```python
from build123d import *

# Parameters (mm, degrees)
SKETCH1_W           = 177.8
SKETCH1_H           = 63.5
SKETCH1_R           = 2.032
BOSS_EXTRUDE1_DEPTH = 6.35
CUT_EXTRUDE1_DEPTH  = 6.35
SKETCH3_R           = 2.413
CUT_EXTRUDE2_DEPTH  = 6.35
LPATTERN1_COUNT     = 3
LPATTERN1_PITCH     = 12.7


with BuildPart() as part:
    # Sketch1 → Boss-Extrude1 (new body)
    with BuildSketch(Plane.XY):
        Rectangle(SKETCH1_W, SKETCH1_H)
        with Locations((-82.804, 25.654)):
            Circle(SKETCH1_R, mode=Mode.SUBTRACT)
        with Locations((-82.804, 0)):
            Circle(SKETCH1_R, mode=Mode.SUBTRACT)
        with Locations((-82.804, -25.654)):
            Circle(SKETCH1_R, mode=Mode.SUBTRACT)
        with Locations((82.804, -25.654)):
            Circle(SKETCH1_R, mode=Mode.SUBTRACT)
        with Locations((82.804, 0)):
            Circle(SKETCH1_R, mode=Mode.SUBTRACT)
        with Locations((82.804, 25.654)):
            Circle(SKETCH1_R, mode=Mode.SUBTRACT)
    extrude(amount=BOSS_EXTRUDE1_DEPTH)

    # Sketch2 → Cut-Extrude1 (cut)
    with BuildSketch(Plane.XY.offset(6.35)):
        Polygon((-75.063183589, 28.589529071), (-75.063183589, -27.290470929), (-51.281087561, -27.290470929), (-50.94437734, 0.649529071), (-50.94437734, 28.589529071), align=None)
        Polygon((-50.94437734, 0.649529071), (-51.281087561, -27.290470929), (-7.031936064, -27.290470929), (-7.031936064, 28.589529071), (-50.94437734, 28.589529071), align=None)
    extrude(amount=-CUT_EXTRUDE1_DEPTH, mode=Mode.SUBTRACT)

    # Sketch3 → Cut-Extrude2 (cut)
    with BuildSketch(Plane.XY.offset(6.35)):
        with Locations((63.5, 19.05)):
            Circle(SKETCH3_R)
    cut_extrude2 = extrude(amount=-CUT_EXTRUDE2_DEPTH, mode=Mode.SUBTRACT)

    # LPattern1: Cut-Extrude2 ×3
    with Locations(*[(0, -i * LPATTERN1_PITCH, 0) for i in range(1, LPATTERN1_COUNT)]):
        add(cut_extrude2, mode=Mode.SUBTRACT)


solid = part.part
```
Geometry: final body of the model. Coordinates: model frame, mm. A direction names the side the tool comes from. Coordinates: 2 decimals unless noted, no trailing zeros. Order: outer loops, then holes, each group sorted by start corner. A loop starts at its lowest first (then second) coordinate and runs counter-clockwise, first axis right, second up. Notation, with made-up numbers: (22.25, -27.75) - (72.25, -27.75) arc R33 cw to (72.25, 3.25) - close; hole circle Ø11 at (0.25, 85.25). An arc over 180 degrees is marked (long way). Write each question's results on one line, items separated by ' | '.
1) Section A-A, the plane y = 19.05. Return loops of the section in (x, z), plus the area to 3 significant figures.
Results list:
outline: (-88.9, 0) - (-75.06, 0) - (-75.06, 6.35) - (-88.9, 6.35) - close; (-7.03, 0) - (61.09, 0) - (61.09, 6.35) - (-7.03, 6.35) - close; (65.91, 0) - (88.9, 0) - (88.9, 6.35) - (65.91, 6.35) - close | area: 666 mm^2
2) Section B-B, the plane x = 63.5. Return loops of the section in (y, z).
Results list:
outline: (-31.75, 0) - (-8.76, 0) - (-8.76, 6.35) - (-31.75, 6.35) - close; (-3.94, 0) - (3.94, 0) - (3.94, 6.35) - (-3.94, 6.35) - close; (8.76, 0) - (16.64, 0) - (16.64, 6.35) - (8.76, 6.35) - close; (21.46, 0) - (31.75, 0) - (31.75, 6.35) - (21.46, 6.35) - close
3) Set-up query: faces 1 (the flat face through (19, 0, 6.35)), 2 (the flat face through (-41, 28.59, 3)). Return all of +Z, -Z, +X, -X, +Y, -Y with unobstructed straight access to the full face (end or side cutting, diameter ignored); none if empty.
Results list:
face 1: +Z, +X, -X, +Y, -Y | face 2: +Z, -Z
4) Pull-direction query (X, two-part tool) for faces 3 (the flat face through (88.9, 0, 3)), 4 (the flat face through (19, 0, 0)), 5 (the flat face through (-88.9, 0, 3)), 6 (the cylindrical face through (61.09, 6.46, 3.22)); classes: pulls with the +X half, pulls with the -X half, needs draft (parallel to the pull), parting line crosses it, or undercut.
Results list:
face 3: pulls with the +X half | face 4: needs draft | face 5: pulls with the -X half | face 6: undercut
5) Line query: line 1 (X direction, y = 19, z = 3.25); line 2 (Y direction, x = 63.5, z = 4.5); line 3 (Y direction, x = -23, z = 1.5). Output: solid intervals per line, ascending. Write a range as from..to.
Results list:
line 1: -88.9..-75.06, -7.03..61.09, 65.91..88.9 | line 2: -31.75..-8.76, -3.94..3.94, 8.76..16.64, 21.46..31.75 | line 3: -31.75..-27.29, 28.59..31.75
6) Section D-D, the plane x = -46. Return loops of the section in (y, z), plus the area to 3 significant figures.
Results list:
outline: (-31.75, 0) - (-27.29, 0) - (-27.29, 6.35) - (-31.75, 6.35) - close; (28.59, 0) - (31.75, 0) - (31.75, 6.35) - (28.59, 6.35) - close | area: 48.4 mm^2
7) Section C-C, the plane y = -15.5. Return loops of the section in (x, z).
Results list:
outline: (-88.9, 0) - (-75.06, 0) - (-75.06, 6.35) - (-88.9, 6.35) - close; (-7.03, 0) - (88.9, 0) - (88.9, 6.35) - (-7.03, 6.35) - close
8) Pin query (flat end, axial travel): pin 1 (4.5 mm diameter, centred on x = 63.5, y = -6.35, fed in from +Z) (1 decimal); pin 2 (6.5 mm diameter, centred on x = -82.804, y = 25.654, fed in from +Z). Return the tip coordinate at first contact, or that it passes through.
Results list:
pin 1: through | pin 2: z = 6.35
